Geometry: final body of the model. Coordinates: model frame, mm. A direction names the side the tool comes from. Coordinates: 2 decimals unless noted, no trailing zeros. Loops run counter-clockwise (first coordinate to the right, second up) from the corner with the lowest first, then second, coordinate; pieces in that order, holes last. Notation, with made-up numbers: (81.5, 87) - (110.5, 87) arc R32 cw to (110.5, 124) - close; hole circle Ø7 at (8, -40). An arc over 180 degrees is marked (long way). Answer in a Markdown table with one row per item.
from build123d import *

# Parameters (mm, degrees)
F0_W     = 2000
F0_H     = 1500
F1_DEPTH = 5
F2_W     = 2000
F2_H     = 400
F3_DEPTH = 10
F5_DEPTH = 10


with BuildPart() as f1:
    # F0 (on Top) → F1 (new body)
    with BuildSketch(Plane.XY):
        with Locations((0, -250)):
            Rectangle(F0_W, F0_H)
    extrude(amount=-F1_DEPTH)

    # F2 (on face) → F3 (join)
    with BuildSketch(Plane(origin=(0, 0, -5), x_dir=(1, 0, 0), z_dir=(0, 0, -1))):
        with Locations((0, 800)):
            Rectangle(F2_W, F2_H)
    extrude(amount=F3_DEPTH)

    # F4 (on Right) → F5 (join)
    with BuildSketch(Plane.YZ):
        Polygon((-600, -15), (-860, -15), (-840, -152.4), (500, -5), (-600, -5), align=None)
    extrude(amount=F5_DEPTH)


solid = f1.part
(1) Cut plane C-C on y = -787. Output: boundary loops of the cut face in (x, z), then the cut area to 3 significant figures.
Verdict:
| item | result |
|---|---|
| outline | (-1000, -15) - (0, -15) - (0, -146.57) - (10, -146.57) - (10, -15) - (1000, -15) - (1000, 0) - (-1000, 0) - close |
| area | 31,300 mm² |
(2) Cut plane A-A on y = -131. Output: boundary loops of the cut face in (x, z).
Verdict:
| item | result |
|---|---|
| outline | (-1000, -5) - (0, -5) - (0, -74.41) - (10, -74.41) - (10, -5) - (1000, -5) - (1000, 0) - (-1000, 0) - close |
(3) First-contact query: pin 1 Ø4 at (x, y) = (471, -684.5) entering from -Z; pin 2 Ø12 at (x, y) = (737, -397) entering from -Z; pin 3 Ø8 at (x, z) = (-336.5, -11) entering from +Y. Flat tips, straight axial feed; report the tip coordinate or a pass-through.
Verdict:
| item | result |
|---|---|
| pin 1 | stops at z = -15 |
| pin 2 | stops at z = -5 |
| pin 3 | stops at y = -600 |
(4) Ray query, probe 1 along Z at (x, y) = (195, 36); probe 2 along Z at (x, y) = (680.5, -621); probe 3 along X at (y, z) = (-663.5, -67.5). Return the intervals inside material, ascending.
Verdict:
| item | result |
|---|---|
| probe 1 | z = -5 to 0 |
| probe 2 | z = -15 to 0 |
| probe 3 | x = 0 to 10 |
(5) Cut plane B-B on x = -752. Output: boundary loops of the cut face in (y, z).
Verdict:
| item | result |
|---|---|
| outline | (-1000, -15) - (-600, -15) - (-600, -5) - (500, -5) - (500, 0) - (-1000, 0) - close |
(6) Access query for faces 1 (the face through (-507, -42, -5)), 2 (the face through (498, -42, -5)), 3 (the face through (4.93, -179.38, -79.73)). Directions: +Z, -Z, +X, -X, +Y, -Y. A direction counts if a zero-diameter tool reaches every point of the face in a straight line with its end or side. Return the directions, or none.
Verdict:
| item | result |
|---|---|
| face 1 | -Z, -X, +Y |
| face 2 | -Z, +X, +Y |
| face 3 | -Z, +X, -X, +Y |
(7) Cut plane D-D on z = -47. Output: boundary loops of the cut face in (x, y).
Verdict:
| item | result |
|---|---|
| outline | (0, -855.34) - (10, -855.34) - (10, 118.18) - (0, 118.18) - close |
